from build123d import *

# Parameters (mm, degrees)
SKIZZE1_R                            = 12.5
AUFSATZ_LINEAR_AUSTRAGEN1_DEPTH      = 10.8
SKIZZE2_R                            = 6
SCHNITT_LINEAR_AUSTRAGEN1_DEPTH      = 7
SCHNITT_LINEAR_AUSTRAGEN2_DEPTH      = 20.013153342
SCHNITT_LINEAR_AUSTRAGEN2_DEPTH_BACK = 20.013153342
SKIZZE3_R                            = 2.5
VERRUNDUNG1_R                        = 1


with BuildPart() as part:
    # Skizze1 → Aufsatz-Linear austragen1 (new body)
    with BuildSketch(Plane(origin=(0, 0, 0), x_dir=(0, 1, 0), z_dir=(0, 0, 1))):
        with Locations(Location((0, 0, 0), (0, 0, 90))):
            Circle(SKIZZE1_R)
    extrude(amount=AUFSATZ_LINEAR_AUSTRAGEN1_DEPTH)

    # Skizze2 → Schnitt-Linear austragen1 (cut)
    with BuildSketch(Plane.XY.offset(10.8)):
        Circle(SKIZZE2_R)
    extrude(amount=-SCHNITT_LINEAR_AUSTRAGEN1_DEPTH, mode=Mode.SUBTRACT)

    # Skizze3 → Schnitt-Linear austragen2 (cut, two sides: drawn at the far end of the back side and taken through both)
    with BuildSketch(Plane.XY.offset(3.8).offset(-SCHNITT_LINEAR_AUSTRAGEN2_DEPTH_BACK)):
        Circle(SKIZZE3_R)
    extrude(amount=SCHNITT_LINEAR_AUSTRAGEN2_DEPTH + SCHNITT_LINEAR_AUSTRAGEN2_DEPTH_BACK, mode=Mode.SUBTRACT)

    # Verrundung1
    verrundung1_edges = [part.edges().sort_by_distance(p)[0] for p in [
        (12.5, 0, 10.8),
        (-6, 0, 10.8),
    ]]
    fillet(verrundung1_edges, radius=VERRUNDUNG1_R)


solid = part.part
CAD build for the part. Positions are in the model's coordinates, mm. A direction names the side the tool comes from. Give positions to 0.01 mm unless a question says otherwise; leave off trailing zeros. Loops run counter-clockwise (first coordinate to the right, second up) from the corner with the lowest first, then second, coordinate; pieces in that order, holes last. Notation, with made-up numbers: M 5,40.25 L 46,40.25 A21 cw 46,44.25 Z; hole C -18.75,27.25 d8. An arc over 180 degrees is marked long. Answer in a Markdown table with one row per item. Add a question column.
Item 1: Band-saw the part on D-D on z = 6.5. Give the cut face in (x, y), then the cut area to 3 significant figures.
Item 2: Tool access for faces 4 (the face through (-0.54, -2.44, 1.87)), 5 (the face through (-6, 0, 7)): list every direction of +Z, -Z, +X, -X, +Y, -Y with a clear straight run to the whole face (end or side of a thin tool).
Item 3: Band-saw the part on A-A on x = 0. Give the cut face in (y, z), then the cut area to 3 significant figures.
Item 4: Probe probe 1 along Y at (x, z) = (0, 1); probe 2 along Y at (x, z) = (0, 6.1); probe 3 along Z at (x, y) = (-1.75, 4). List the from-to ranges inside material, lowest first.
Item 5: Mould opens along Y. For faces 1 (the face through (0, 8, 10.8)), 2 (the face through (3, 0, 3.8)), 3 (the face through (-11.923, -3.755, 4.831)) say: +Y half, -Y half, draft (parallel to the pull), parting line (faces both ways), or undercut.
Item 6: Drop flat-ended pins along their axis: P1, Ø3, axis at y = -7, z = 5, coming from the +X side (3 decimals); P2, Ø2, axis at x = -9, z = 5, coming from the -Y side; P3, Ø5, axis at x = 5.5, z = 7.5, coming from the +Y side; P4, Ø4, axis at x = 0, y = 0, coming from the -Z side. Give the stop position or say it passes through.
Item 7: Band-saw the part on C-C on z = 3.5. Give the cut face in (x, y).
Reply:
| question | item | result |
|---|---|---|
| 1 | outline | C 0,0 d25; hole C 0,0 d12 |
| 1 | area | 378 mm^2 |
| 2 | face 4 | +Z, -Z |
| 2 | face 5 | +Z |
| 3 | outline | M -12.5,0 L -2.5,0 L -2.5,3.8 L -6,3.8 L -6,9.8 A1 ccw -7,10.8 L -11.5,10.8 A1 ccw -12.5,9.8 Z; M 2.5,0 L 12.5,0 L 12.5,9.8 A1 ccw 11.5,10.8 L 7,10.8 A1 ccw 6,9.8 L 6,3.8 L 2.5,3.8 Z |
| 3 | area | 166 mm^2 |
| 4 | probe 1 | y = -12.5 to -2.5, 2.5 to 12.5 |
| 4 | probe 2 | y = -12.5 to -6, 6 to 12.5 |
| 4 | probe 3 | z = 0 to 3.8 |
| 5 | face 1 | draft |
| 5 | face 2 | undercut |
| 5 | face 3 | parting line |
| 6 | P1 | stops at x = 11.225 |
| 6 | P2 | stops at y = -9.6 |
| 6 | P3 | stops at y = 12.13 |
| 6 | P4 | passes through |
| 7 | outline | C 0,0 d25; hole C 0,0 d5 |
